Check sheet for the modelled part. Datum: model origin and axes. Units: mm. Face numbers are marked on the shaded views. A direction names the side the tool comes from. Round coordinates to 2 decimals unless told otherwise and drop trailing zeros. Write each loop counter-clockwise with the first axis right and the second up, starting at its lowest first coordinate (ties: lowest second). Pieces come first, ordered by that corner, then holes. Notation, with made-up numbers: M -15.75,33.25 L 37.25,33.25 A35 ccw 37.25,72.25 Z; hole C -20,29 d6. An arc over 180 degrees is marked long. One line per item, written item: value.
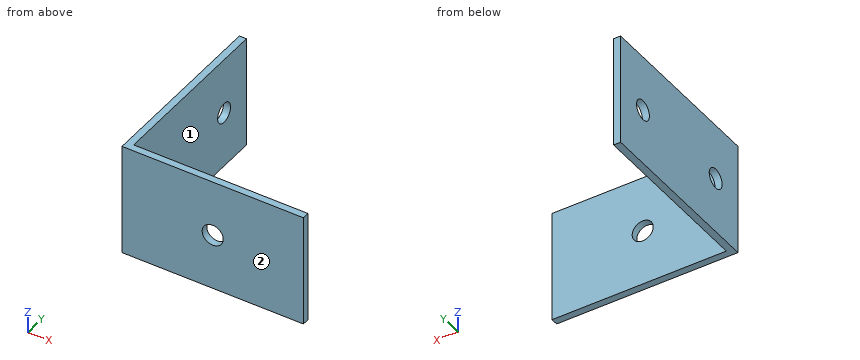
from build123d import *

# Parameters (mm, degrees)
F1_DEPTH = 25.4
F2_R     = 2.25
F3_DEPTH = 41.001
F4_R     = 2.38125
F5_DEPTH = 41.001


with BuildPart() as f1:
    # F0 (on Top) → F1 (new body)
    with BuildSketch(Plane.XY):
        Polygon((-29.149991, 41), (-30.749991, 41), (-30.749991, 0), (10.250009, 0), (10.250009, 1.6), (-29.149991, 1.6), align=None)
    extrude(amount=F1_DEPTH)

    # F2 (on face) → F3 (cut, through all)
    with BuildSketch(Plane(origin=(-30.749991, 0, 0), x_dir=(0, -1, 0), z_dir=(-1, 0, 0))):
        with Locations((-33.2, 12.7)):
            Circle(F2_R)
        with Locations((-7.8, 12.7)):
            Circle(F2_R)
    extrude(amount=-F3_DEPTH, mode=Mode.SUBTRACT)

    # F4 (on face) → F5 (cut, through all)
    with BuildSketch(Plane.XZ):
        with Locations((-10.249991, 12.7)):
            Circle(F4_R)
    extrude(amount=-F5_DEPTH, mode=Mode.SUBTRACT)


solid = f1.part
Q1. Access from +Z, -Z, +X, -X, +Y, -Y to the whole of each face (thin tool, end or side, straight path). Record for the marked faces 1 and 2.
Completed:
face 1: +Z, -Z, +X, +Y
face 2: +Z, -Z, +X, -X, -Y
Q2. Depth check by flat-ended pin: P1, Ø8, axis at x = -11.5, z = 20, coming from the +Y side; P2, Ø3, axis at x = -10.25, z = 12.7, coming from the +Y side; P3, Ø6, axis at y = 18, z = 12, coming from the +X side; P4, Ø8, axis at x = 2.5, z = 8, coming from the -Y side. Enter the tip coordinate at first touch or a pass-through.
Completed:
P1: y = 1.6
P2: through
P3: x = -29.15
P4: y = 0
Q3. Sectioned sample at A-A on y = 7.8. Enter the section's corners in (x, z), and give its area (3 significant figures).
Completed:
outline: M -30.75,0 L -29.15,0 L -29.15,10.45 L -30.75,10.45 Z; M -30.75,14.95 L -29.15,14.95 L -29.15,25.4 L -30.75,25.4 Z
area: 33.4 mm^2
Q4. Sectioned sample at D-D on z = 19.25. Enter the section's corners in (x, y), and give its area (3 significant figures).
Completed:
outline: M -30.75,0 L 10.25,0 L 10.25,1.6 L -29.15,1.6 L -29.15,41 L -30.75,41 Z
area: 129 mm^2
Q5. Sectioned sample at B-B on z = 12.7. Enter the section's corners in (x, y).
Completed:
outline: M -30.75,0 L -12.63,0 L -12.63,1.6 L -29.15,1.6 L -29.15,5.55 L -30.75,5.55 Z; M -30.75,10.05 L -29.15,10.05 L -29.15,30.95 L -30.75,30.95 Z; M -30.75,35.45 L -29.15,35.45 L -29.15,41 L -30.75,41 Z; M -7.87,0 L 10.25,0 L 10.25,1.6 L -7.87,1.6 Z
Q6. Sectioned sample at C-C on x = -11. Enter the section's corners in (y, z), and give its area (3 significant figures).
Completed:
outline: M 0,0 L 1.6,0 L 1.6,10.44 L 0,10.44 Z; M 0,14.96 L 1.6,14.96 L 1.6,25.4 L 0,25.4 Z
area: 33.4 mm^2
Q7. Scan lines: line 1 (Z direction, x = -29.7, y = 7.8); line 2 (Y direction, x = 6, z = 3.5); line 3 (X direction, y = 3.5, z = 7.75). Record each from-to range of solid material in increasing order. Write a range as [from, to].
Completed:
line 1: [0, 10.45], [14.95, 25.4]
line 2: [0, 1.6]
line 3: [-30.75, -29.15]
